Verification items for the finished model (mm, model axes). A direction names the side the tool comes from. Coordinates: 2 decimals unless noted, no trailing zeros. Write each loop counter-clockwise with the first axis right and the second up, starting at its lowest first coordinate (ties: lowest second). Pieces come first, ordered by that corner, then holes. Notation, with made-up numbers: M -28.5,69.5 L 21.5,69.5 A33 cw 21.5,108.5 Z; hole C -17.5,-12 d9. An arc over 180 degrees is marked long. One line per item, written item: value.
```python
from build123d import *

# Parameters (mm, degrees)
SKETCH1_W                = 57
SKETCH1_H                = 57
EXTRUDE1_DEPTH           = 76
F_5_0_5_DIAMETER_HOLE1_D = 5
SKETCH6_R                = 4
SKETCH6_R_2              = 2.5
EXTRUDE4_DEPTH           = 71
FILLET1_R                = 5
SKETCH7_R                = 3
EXTRUDE5_DEPTH           = 101
SKETCH8_R                = 15
EXTRUDE6_DEPTH           = 3
FILLET2_R                = 1
SKETCH9_R                = 5.5
BOSS_EXTRUDE1_DEPTH      = 174
CHAMFER1_SIZE            = 0.5
SKETCH10_R               = 4
BOSS_EXTRUDE2_DEPTH      = 10
CHAMFER2_SIZE            = 0.5
CUT_EXTRUDE1_REACH       = 196.724
SKETCH11_W               = 136.965596246
SKETCH11_H               = 58.892429462
FILLET3_R                = 1


with BuildPart() as part:
    # Sketch1 → Extrude1 (new body)
    with BuildSketch(Plane(origin=(0, 0, 0), x_dir=(1, 0, 0), z_dir=(0, 1, 0))):
        Rectangle(SKETCH1_W, SKETCH1_H)
    extrude(amount=EXTRUDE1_DEPTH)

    # Ø5.0 (5) Diameter Hole1 (through all)
    with Locations(Plane.XZ):
        with Locations((-23.5, 23.5), (23.5, 23.5), (23.5, -23.5), (-23.5, -23.5)):
            Hole(F_5_0_5_DIAMETER_HOLE1_D / 2)

    # Sketch6 → Extrude4 (cut)
    # profile 1 of 12: a face of its own
    with BuildSketch(Plane(origin=(0, 76, 0), x_dir=(1, 0, 0), z_dir=(0, 1, 0))):
        Polygon((-28.5, 28.5), (-19.5, 28.5), (-19.5, 32.511741208), (-33.908905561, 32.511741208), (-33.908905561, 19.5), (-28.5, 19.5), align=None)
    # profile 2 of 12: a face of its own
    with BuildSketch(Plane(origin=(0, 76, 0), x_dir=(1, 0, 0), z_dir=(0, 1, 0))):
        with BuildLine():
            ThreePointArc((-23.5, 19.5), (-26.328427125, 26.328427125), (-19.5, 23.5))
            Line((-19.5, 23.5), (-19.5, 28.5))
            Line((-19.5, 28.5), (-28.5, 28.5))
            Line((-28.5, 28.5), (-28.5, 19.5))
            Line((-28.5, 19.5), (-23.5, 19.5))
        make_face()
    # profile 3 of 12: a face of its own
    with BuildSketch(Plane(origin=(0, 76, 0), x_dir=(1, 0, 0), z_dir=(0, 1, 0))):
        with Locations((-23.5, 23.5)):
            Circle(SKETCH6_R)
        with Locations(Location((-23.5, 23.5, 0), (0, 0, 90))):
            Circle(SKETCH6_R_2, mode=Mode.SUBTRACT)
    # profile 4 of 12: a face of its own
    with BuildSketch(Plane(origin=(0, 76, 0), x_dir=(1, 0, 0), z_dir=(0, 1, 0))):
        Polygon((19.5, 36.471560472), (19.5, 28.5), (28.5, 28.5), (28.5, 19.5), (41.168352552, 19.5), (41.168352552, 36.471560472), align=None)
    # profile 5 of 12: a face of its own
    with BuildSketch(Plane(origin=(0, 76, 0), x_dir=(1, 0, 0), z_dir=(0, 1, 0))):
        with BuildLine():
            Line((28.5, 28.5), (19.5, 28.5))
            Line((19.5, 28.5), (19.5, 23.5))
            ThreePointArc((19.5, 23.5), (23.5, 27.5), (27.5, 23.5))
            ThreePointArc((27.5, 23.5), (26.328427125, 20.671572875), (23.5, 19.5))
            Line((23.5, 19.5), (28.5, 19.5))
            Line((28.5, 19.5), (28.5, 28.5))
        make_face()
    # profile 6 of 12: a face of its own
    with BuildSketch(Plane(origin=(0, 76, 0), x_dir=(1, 0, 0), z_dir=(0, 1, 0))):
        with Locations((23.5, 23.5)):
            Circle(SKETCH6_R)
        with Locations(Location((23.5, 23.5, 0), (0, 0, 90))):
            Circle(SKETCH6_R_2, mode=Mode.SUBTRACT)
    # profile 7 of 12: a face of its own
    with BuildSketch(Plane(origin=(0, 76, 0), x_dir=(1, 0, 0), z_dir=(0, 1, 0))):
        with Locations((23.5, -23.5)):
            Circle(SKETCH6_R)
        with Locations(Location((23.5, -23.5, 0), (0, 0, 90))):
            Circle(SKETCH6_R_2, mode=Mode.SUBTRACT)
    # profile 8 of 12: a face of its own
    with BuildSketch(Plane(origin=(0, 76, 0), x_dir=(1, 0, 0), z_dir=(0, 1, 0))):
        with BuildLine():
            Line((28.5, -28.5), (28.5, -19.5))
            Line((28.5, -19.5), (23.5, -19.5))
            ThreePointArc((23.5, -19.5), (26.328427125, -20.671572875), (27.5, -23.5))
            ThreePointArc((27.5, -23.5), (23.5, -27.5), (19.5, -23.5))
            Line((19.5, -23.5), (19.5, -28.5))
            Line((19.5, -28.5), (28.5, -28.5))
        make_face()
    # profile 9 of 12: a face of its own
    with BuildSketch(Plane(origin=(0, 76, 0), x_dir=(1, 0, 0), z_dir=(0, 1, 0))):
        Polygon((44.252209519, -19.5), (28.5, -19.5), (28.5, -28.5), (19.5, -28.5), (19.5, -40.050429997), (44.252209519, -40.050429997), align=None)
    # profile 10 of 12: a face of its own
    with BuildSketch(Plane(origin=(0, 76, 0), x_dir=(1, 0, 0), z_dir=(0, 1, 0))):
        Polygon((-28.5, -28.5), (-28.5, -19.5), (-37.670786859, -19.5), (-37.670786859, -37.828231874), (-19.5, -37.828231874), (-19.5, -28.5), align=None)
    # profile 11 of 12: a face of its own
    with BuildSketch(Plane(origin=(0, 76, 0), x_dir=(1, 0, 0), z_dir=(0, 1, 0))):
        with BuildLine():
            Line((-23.5, -19.5), (-28.5, -19.5))
            Line((-28.5, -19.5), (-28.5, -28.5))
            Line((-28.5, -28.5), (-19.5, -28.5))
            Line((-19.5, -28.5), (-19.5, -23.5))
            ThreePointArc((-19.5, -23.5), (-26.328427125, -26.328427125), (-23.5, -19.5))
        make_face()
    # profile 12 of 12: a face of its own
    with BuildSketch(Plane(origin=(0, 76, 0), x_dir=(1, 0, 0), z_dir=(0, 1, 0))):
        with Locations((-23.5, -23.5)):
            Circle(SKETCH6_R)
        with Locations(Location((-23.5, -23.5, 0), (0, 0, 90))):
            Circle(SKETCH6_R_2, mode=Mode.SUBTRACT)
    extrude(amount=-EXTRUDE4_DEPTH, mode=Mode.SUBTRACT)

    # Fillet1
    fillet1_edges = [part.edges().sort_by_distance(p)[0] for p in [
        (-28.5, 2.5, 28.5),
        (-28.5, 2.5, -28.5),
        (28.5, 2.5, -28.5),
        (28.5, 2.5, 28.5),
    ]]
    fillet(fillet1_edges, radius=FILLET1_R)



with BuildPart() as body_2:
    # Sketch7 → Extrude5 (new body)
    with BuildSketch(Plane(origin=(0, 76, 0), x_dir=(1, 0, 0), z_dir=(0, 1, 0))):
        with Locations(Location((0, 0, 0), (0, 0, 270))):
            Circle(SKETCH7_R)
    extrude(amount=-EXTRUDE5_DEPTH)


with BuildPart() as part_1:
    add(part.part)

    add(body_2.part)  # Extrude6 merges body 2
    # Sketch8 → Extrude6 (add)
    with BuildSketch(Plane.XZ):
        with Locations(Location((0, 0, 0), (0, 0, 270))):
            Circle(SKETCH8_R)
    extrude(amount=EXTRUDE6_DEPTH)

    # Fillet2
    fillet2_edges = [part_1.edges().sort_by_distance(p)[0] for p in [
        (-28.5, 40.5, 19.5),
        (0, 76, 28.5),
        (-19.5, 40.5, 28.5),
        (-19.5, 76, 26),
        (-20.671572875, 76, 20.671572875),
        (-26, 76, 19.5),
        (-28.5, 76, 0),
        (-28.5, 40.5, -19.5),
        (-19.5, 40.5, -28.5),
        (-19.5, 76, -26),
        (-26, 76, -19.5),
        (-20.671572875, 76, -20.671572875),
        (0, 76, -28.5),
        (19.5, 76, -26),
        (26, 76, -19.5),
        (20.671572875, 76, -20.671572875),
        (19.5, 40.5, -28.5),
        (28.5, 40.5, -19.5),
        (19.5, 40.5, 28.5),
        (28.5, 76, 0),
        (26, 76, 19.5),
        (19.5, 76, 26),
        (20.671572875, 76, 20.671572875),
        (28.5, 40.5, 19.5),
    ]]
    fillet(fillet2_edges, radius=FILLET2_R)

    # Sketch9 → Boss-Extrude1 (add)
    with BuildSketch(Plane.XZ):
        with Locations(Location((0, 0, 0), (0, 0, 270))):
            Circle(SKETCH9_R)
    extrude(amount=BOSS_EXTRUDE1_DEPTH)

    # Chamfer1
    chamfer1_edges = [part_1.edges().sort_by_distance(p)[0] for p in [
        (0, -174, 5.5),
    ]]
    chamfer(chamfer1_edges, length=CHAMFER1_SIZE)

    # Sketch10 → Boss-Extrude2 (add)
    with BuildSketch(Plane.XZ.offset(174)):
        with Locations(Location((0, 0, 0), (0, 0, 270))):
            Circle(SKETCH10_R)
    extrude(amount=BOSS_EXTRUDE2_DEPTH)

    # Chamfer2
    chamfer2_edges = [part_1.edges().sort_by_distance(p)[0] for p in [
        (0, -184, 4),
    ]]
    chamfer(chamfer2_edges, length=CHAMFER2_SIZE)

    # Sketch11 → Cut-Extrude1 (cut, up to next)
    with BuildSketch(Plane.XY.offset(28.5), mode=Mode.PRIVATE) as cut_extrude1_sk1:
        with Locations((0.168266434, 85.446214731)):
            Rectangle(SKETCH11_W, SKETCH11_H)
    cut_extrude1_tool1 = extrude(cut_extrude1_sk1.sketch, amount=-CUT_EXTRUDE1_REACH, mode=Mode.PRIVATE) & part_1.part
    add(cut_extrude1_tool1.solids().sort_by_distance((0.168266, 85.446215, 28.5))[0], mode=Mode.SUBTRACT)

    # Fillet3
    fillet3_edges = [part_1.edges().sort_by_distance(p)[0] for p in [
        (0, 56, 28.5),
        (19.5, 56, 25.5),
        (19.207106781, 56, 28.207106781),
        (-19.207106781, 56, 28.207106781),
        (-28.207106781, 56, 19.207106781),
        (-28.207106781, 56, -19.207106781),
        (-19.207106781, 56, -28.207106781),
        (19.207106781, 56, -28.207106781),
        (19.5, 56, -25.5),
        (25.5, 56, -19.5),
        (28.207106781, 56, -19.207106781),
        (28.207106781, 56, 19.207106781),
        (25.5, 56, 19.5),
        (28.5, 56, 0),
        (0, 56, -28.5),
        (-28.5, 56, 0),
        (-25.5, 56, -19.5),
        (-19.5, 56, -25.5),
        (-20.671572875, 56, -20.671572875),
        (20.671572875, 56, -20.671572875),
        (20.671572875, 56, 20.671572875),
        (-19.5, 56, 25.5),
        (-25.5, 56, 19.5),
        (-20.671572875, 56, 20.671572875),
    ]]
    fillet(fillet3_edges, radius=FILLET3_R)


solid = part_1.part
```
Item 1: Scan lines: line 1 (Z direction, x = -23.5, y = 2.2); line 2 (X direction, y = 1, z = -23); line 3 (Z direction, x = 23, y = 36.5). Record each from-to range of solid material in increasing order.
The answers:
line 1: z = -28.5 to -26, -21 to 21, 26 to 28.5
line 2: x = -28.5 to -25.95, -21.05 to 21.05, 25.95 to 28.5
line 3: z = -19.53 to 19.53
Item 2: Access from +Z, -Z, +X, -X, +Y, -Y to the whole of each face (thin tool, end or side, straight path). Record for faces 5 (the face through (-19.5, 30, 26)), 6 (the face through (-21.66, 2.53, 25.19)), 7 (the face through (20.703, 30.35, 20.641)), 8 (the face through (-19.5, 30, -25)).
The answers:
face 5: +Z, -X, +Y
face 6: +Y, -Y
face 7: +Z, +X, +Y
face 8: -Z, -X, +Y
Item 3: Go/stop test with flat-tipped pins: P1, Ø5, axis at x = -1, z = -22, coming from the -Y side; P2, Ø24, axis at x = -5, z = 1.5, coming from the -Y side; P3, Ø4, axis at x = 23.5, z = 23.5, coming from the +Y side; P4, Ø1.2, axis at y = 22.5, z = -25, coming from the +X side. Record where each tip stops, or that it passes through.
The answers:
P1: stops at y = 0
P2: stops at y = -184
P3: passes through
P4: stops at x = 19.5
Item 4: Cross-section at A-A, the plane x = 8.5. Enter the section's corners in (y, z).
The answers:
outline: M -3,-12.36 L 0,-12.36 L 0,-28.5 L 55,-28.5 A1 ccw 56,-27.5 L 56,27.5 A1 ccw 55,28.5 L 0,28.5 L 0,12.36 L -3,12.36 Z
Item 5: Draft check along Z on faces 1 (the face through (25.34, 2.53, 25.19)), 2 (the face through (25, 30, -19.5)), 3 (the face through (25, 5, -26)), 4 (the face through (0, 27, 28.5)). Enter one of: released by +Z, released by -Z, zero draft, split by the parting line, or undercut.
The answers:
face 1: undercut
face 2: released by -Z
face 3: zero draft
face 4: released by +Z
Item 6: Cross-section at B-B, the plane y = -136. Enter the section's corners in (x, z).
The answers:
outline: C 0,0 d11
